Autodesk Inventor part; units mm, degrees
ref_plane "YZ Plane" through (0, 0, 0) normal (1, 0, 0) x (0, 1, 0)
ref_plane "XZ Plane" through (0, 0, 0) normal (0, 1, 0) x (-1, 0, 0)
ref_plane "XY Plane" through (0, 0, 0) normal (0, 0, 1) x (1, 0, 0)
sketch "Sketch1" plane through (0, 0, 0) normal (1, 0, 0) x (0, 1, 0)
  line L0 (0, 0) -> (0, -60)
  line L1 (0, -60) -> (45, -60)
  line L2 (45, -60) -> (45, -40)
  line L3 (45, -40) -> (30, -40)
  line L4 (30, -40) -> (30, -20)
  line L5 (30, -20) -> (15, -20)
  line L6 (15, -20) -> (15, 0)
  line L7 (15, 0) -> (0, 0)
  dimension "d0" = 60
  dimension "d1" = 45
  dimension "d2" = 20
  dimension "d3" = 15
  dimension "d4" = 15
  dimension "d5" = 20
extrude "Extrusion1" add sketch "Sketch1" along normal mid plane 25
fillet "Fillet1" radius 15 1 edges at (0, 0, -60)
Geometry: final body of the model. Coordinates: model frame, mm. A direction names the side the tool comes from. Coordinates: 2 decimals unless noted, no trailing zeros. Loops run counter-clockwise (first coordinate to the right, second up) from the corner with the lowest first, then second, coordinate; pieces in that order, holes last. Notation, with made-up numbers: M 5.25,18.5 L 53.25,18.5 A8 ccw 53.25,28.5 Z; hole C 59,51.5 d5. An arc over 180 degrees is marked long. One line per item, written item: value. Start each with the question number.
1) Reachability of faces 1 (the flat face through (0, 15, -10)), 2 (the flat face through (-12.5, 17, -36)) from +Z, -Z, +X, -X, +Y, -Y: full face, straight path, thin tool, end or side. Return the list, or none.
2) Material intervals for L1, parallel to Y at x = -6.75, z = -39; L2, parallel to Z at x = -10.5, y = 27.5; L3, parallel to Y at x = 4, z = -16, sorted ascending. Write a range as from..to.
3) Cut plane A-A (x = 9). Return loops of the section in (y, z), then the cut area to 3 significant figures.
4) Cut plane C-C (z = -28.5). Return loops of the section in (x, y).
5) Cut plane B-B (y = 22.5). Return loops of the section in (x, z).
6) Pin query (flat end, axial travel): P1, Ø2, axis at x = -5.5, y = 11.5, coming from the -Z side; P2, Ø10, axis at x = 0, y = 8, coming from the +Z side; P3, Ø3, axis at x = 8, z = -23, coming from the +Y side; P4, Ø4, axis at x = 8, y = 24.5, coming from the +Z side. Return the tip coordinate at first contact, or that it passes through.
Evaluation:
1. face 1: +Z, +X, -X, +Y
1. face 2: +Z, -Z, -X, +Y, -Y
2. L1: 0..30
2. L2: -60..-20
2. L3: 0..15
3. outline: M 0,-45 A15 ccw 15,-60 L 45,-60 L 45,-40 L 30,-40 L 30,-20 L 15,-20 L 15,0 L 0,0 Z
3. area: 1,750 mm^2
4. outline: M -12.5,0 L 12.5,0 L 12.5,30 L -12.5,30 Z
5. outline: M -12.5,-60 L 12.5,-60 L 12.5,-20 L -12.5,-20 Z
6. P1: z = -59.79
6. P2: z = 0
6. P3: y = 30
6. P4: z = -20
